Read the model definition and answer for the solid it produces. Units are mm, in the model's axes. Face numbers are marked on the shaded views. A direction names the side the tool comes from. Round coordinates to 2 decimals unless told otherwise and drop trailing zeros. Loops run counter-clockwise (first coordinate to the right, second up) from the corner with the lowest first, then second, coordinate; pieces in that order, holes last. Notation, with made-up numbers: (53.25, -21) - (75.25, -21) arc R12 cw to (75.25, 1) - close; hole circle Ø9 at (-12, 56). An arc over 180 degrees is marked (long way). Answer as CSV lines item,"result".
```python
from build123d import *

# Parameters (mm, degrees)
F0_W         = 9.525
F0_H         = 9.525
F1_DEPTH     = 2.286
F2_T1_DEPTH  = 21.3619144247
F3_W         = 2.9083
F3_H         = 9.525
F3_W_2       = 6.8834
F4_DEPTH     = 1.905
F5_R         = 1.6556676611
F6_W         = 12.7
F6_H         = 1.27
F7_DEPTH     = 3.937
F8_SIZE2     = 8.7232408068
F8_SIZE      = 3.175
F9_T4_DEPTH  = 12.7
F9_T9_DEPTH  = 12.7
F10_T1_DEPTH = 20.3689561099


# Not quite as in the source:
# - a fillet or chamfer that OpenCascade refuses, or shapes differently, is made with other operations: its cross-section is extruded or revolved along the edge and cut away or added


with BuildPart() as f1:
    # F0 (on Top) → F1 (new body)
    with BuildSketch(Plane.XY):
        Rectangle(F0_W, F0_H)
    extrude(amount=F1_DEPTH)

    # F2: chamfer of 1.3208 x 2.2876927066 on 2 edges, made by hand

    # F2_s2 → F2_t1 (cut)
    with BuildSketch(Plane.XZ.offset(-10.6809572123)):
        Polygon((-4.7625, -0.0016927066), (-3.4417, 2.286), (-4.7625, 2.286), align=None)
        Polygon((4.7625, -0.0016927066), (3.4417, 2.286), (4.7625, 2.286), align=None)
    extrude(amount=F2_T1_DEPTH, mode=Mode.SUBTRACT)

    # F3 (on face) → F4 (join)
    with BuildSketch(Plane.XY.offset(2.286)):
        with Locations((4.89585, 0)):
            Rectangle(F3_W, F3_H)
        Rectangle(F3_W_2, F3_H)
        with Locations((-4.89585, 0)):
            Rectangle(F3_W, F3_H)
    extrude(amount=F4_DEPTH)

    # F5
    f5_edges = [f1.edges().sort_by_distance(p)[0] for p in [
        (0, 4.7625, 4.191),
        (0, -4.7625, 4.191),
    ]]
    fillet(f5_edges, radius=F5_R)

    # F6 (on face) → F7 (join)
    with BuildSketch(Plane.XY.offset(4.191)):
        Rectangle(F6_W, F6_H)
    extrude(amount=F7_DEPTH)

    # F8
    f8_edges = [f1.edges().sort_by_distance(p)[0] for p in [
        (-6.35, 0, 8.128),
    ]]
    f8_side = f1.faces().sort_by_distance((-6.35, 0, 3.872106))[0]
    chamfer(f8_edges, length=F8_SIZE, length2=F8_SIZE2, reference=f8_side)

    # F9: fillet of radius 2.8207671263 on 2 edges, made by hand


with BuildPart() as f9_tool2:
    # F9_s3 → F9_t4 (new body)
    with BuildSketch(Plane.YZ.offset(-6.35)):
        with BuildLine():
            ThreePointArc((-0.635, 6.9981468006), (-1.3849039981, 5.0828783899), (-3.235890411, 4.1859623453))
            Line((-3.235890411, 4.1859623453), (-3.2139027394, 3.9047438998))
            ThreePointArc((-3.2139027394, 3.9047438998), (-3.1068323389, 3.9089232874), (-0.635, 3.9089232874))
            Line((-0.635, 3.9089232874), (-0.3529232874, 4.191))
            Line((-0.3529232874, 4.191), (-0.3529232874, 6.9981468006))
            Line((-0.3529232874, 6.9981468006), (-0.635, 6.9981468006))
        make_face()
    extrude(amount=F9_T4_DEPTH)

    split(bisect_by=Plane(origin=(-2.3346724085, 0, 6.4144597241), x_dir=(0, 1, 0), z_dir=(0.3420201433, 0, -0.9396926208)), keep=Keep.TOP)


with BuildPart() as f1_1:
    add(f1.part)

    # F9_t1: union F9_tool2
    add(f9_tool2.part)


with BuildPart() as f9_tool7:
    # F9_s8 → F9_t9 (new body)
    with BuildSketch(Plane.YZ.offset(6.35)):
        with BuildLine():
            ThreePointArc((0.635, 6.9981468006), (1.3849039981, 5.0828783899), (3.235890411, 4.1859623453))
            Line((3.235890411, 4.1859623453), (3.2139027394, 3.9047438998))
            ThreePointArc((3.2139027394, 3.9047438998), (3.1068323389, 3.9089232874), (0.635, 3.9089232874))
            Line((0.635, 3.9089232874), (0.3529232874, 4.191))
            Line((0.3529232874, 4.191), (0.3529232874, 6.9981468006))
            Line((0.3529232874, 6.9981468006), (0.635, 6.9981468006))
        make_face()
    extrude(amount=-F9_T9_DEPTH)

    split(bisect_by=Plane(origin=(-2.3346724085, 0, 6.4144597241), x_dir=(0, 1, 0), z_dir=(0.3420201433, 0, -0.9396926208)), keep=Keep.TOP)


with BuildPart() as f1_2:
    add(f1_1.part)

    # F9_t6: union F9_tool7
    add(f9_tool7.part)

    # F10: fillet of radius 5.08 on 1 edges, made by hand

    # F10_s2 → F10_t1 (cut)
    with BuildSketch(Plane.XZ.offset(-10.184478055)):
        with BuildLine():
            ThreePointArc((-6.3503933611, 2.2860725742), (-5.2327762913, 4.646139378), (-3.0907506998, 6.1396954024))
            Line((-3.0907506998, 6.1396954024), (-3.2645725807, 6.6172670953))
            ThreePointArc((-3.2645725807, 6.6172670953), (-4.8941288268, 6.0237314555), (-6.5238218809, 5.4305716928))
            Line((-6.5238218809, 5.4305716928), (-6.8582211803, 4.953))
            ThreePointArc((-6.8582211803, 4.953), (-6.8582211803, 3.6195362871), (-6.8501795082, 2.3782819842))
            Line((-6.8501795082, 2.3782819842), (-6.3503933611, 2.2860725742))
        make_face()
    extrude(amount=F10_T1_DEPTH, mode=Mode.SUBTRACT)


solid = f1_2.part
```
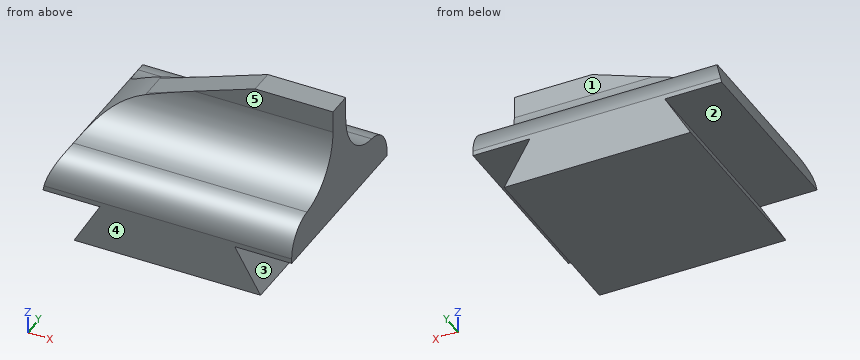
1) Each of these flat-tipped pins is pushed along its axis until it touches: P1, Ø0.9, axis at x = 1.5, z = 7.5, coming from the +Y side (3 decimals); P2, Ø1, axis at x = -1, z = 4, coming from the +Y side. Where does it stop, or does it pass through?
Entries:
P1,"stops at y = 0.635"
P2,"stops at y = 4.45"
2) A cutting plane is placed at A-A, the plane x = -4. Determine the outline of the cut face in (y, z).
Entries:
outline,"(-4.76, 0) - (4.76, 0) - (4.76, 1.32) - (-4.76, 1.32) - close; (-4.76, 2.29) - (4.76, 2.29) - (4.76, 2.54) arc R1.66 ccw to (3.24, 4.19) arc R2.82 cw to (0.95, 5.7) - (-0.95, 5.7) arc R2.82 cw to (-3.24, 4.19) arc R1.66 ccw to (-4.76, 2.54) - close"
3) Find the intervals of material crossed by line 1 (Z direction, x = 1.75, y = 3.25); line 2 (Z direction, x = 4, y = -1.25); line 3 (Z direction, x = 4.25, y = -4.25), in increasing order.
Entries:
line 1,"z = 0 to 4.18"
line 2,"z = 0 to 1.32, 2.29 to 5.24"
line 3,"z = 0 to 0.89, 2.29 to 3.73"
4) A tool of negligible diameter and unlimited length cuts with its end or side. For the marked faces 1, 2, 3, 4 and 5, from which of +Z, -Z, +X, -X, +Y, -Y can it reach the whole face along a straight path? Write none if from no direction.
Entries:
face 1,"+Z, +X, -X, +Y"
face 2,"-X, +Y, -Y"
face 3,"+X, +Y, -Y"
face 4,"+Z, -Z, +X, -X, -Y"
face 5,"+Z, +X, -X, -Y"
5) A cutting plane is placed at D-D, the plane z = 5.5. Determine the outline of the cut face in (x, y).
Entries:
outline,"(-4.31, -1.07) - (6.35, -1.07) - (6.35, 1.07) - (-4.31, 1.07) - close"
6) A cutting plane is placed at C-C, the plane x = -1. Determine the outline of the cut face in (y, z) (1 decimal), plus the area to 3 significant figures.
Entries:
outline,"(-4.8, 0) - (4.8, 0) - (4.8, 2.5) arc R1.7 ccw to (3.2, 4.2) arc R2.8 cw to (0.6, 6.9) - (-0.6, 6.9) arc R2.8 cw to (-3.2, 4.2) arc R1.7 ccw to (-4.8, 2.5) - close"
area,"45.5 mm^2"
